from build123d import *

# Parameters (mm, degrees)
F0_W     = 508
F0_H     = 622.3
F0_W_2   = 68
F0_H_2   = 50.8
F1_DEPTH = 25.4
F2_DEPTH = 12.7
F3_DEPTH = 6.35


with BuildPart() as f1:
    # F0 (on Front) → F1 (new body)
    with BuildSketch(Plane.XZ):
        with Locations((0, -2.179809)):
            Rectangle(F0_W, F0_H)
        with BuildLine():
            Line((-44.45, 99.420191), (-44.45, 137.520191))
            Line((-44.45, 137.520191), (44.45, 137.520191))
            Line((44.45, 137.520191), (44.45, 99.420191))
            Line((44.45, 99.420191), (25.4, 99.420191))
            ThreePointArc((25.4, 99.420191), (20.909872, 97.560319), (19.05, 93.070191))
            Line((19.05, 93.070191), (19.05, 42.270191))
            ThreePointArc((19.05, 42.270191), (20.909872, 37.780063), (25.4, 35.920191))
            Line((25.4, 35.920191), (44.45, 35.920191))
            Line((44.45, 35.920191), (44.45, -2.179809))
            Line((44.45, -2.179809), (-44.45, -2.179809))
            Line((-44.45, -2.179809), (-44.45, 35.920191))
            Line((-44.45, 35.920191), (-25.4, 35.920191))
            ThreePointArc((-25.4, 35.920191), (-20.909872, 37.780063), (-19.05, 42.270191))
            Line((-19.05, 42.270191), (-19.05, 93.070191))
            ThreePointArc((-19.05, 93.070191), (-20.909872, 97.560319), (-25.4, 99.420191))
            Line((-25.4, 99.420191), (-44.45, 99.420191))
        make_face(mode=Mode.SUBTRACT)
        with Locations((0.576081, 175.620191)):
            Rectangle(F0_W_2, F0_H_2, mode=Mode.SUBTRACT)
    extrude(amount=F1_DEPTH)

    # F0 (on Front) → F2 (join)
    with BuildSketch(Plane.XZ):
        with Locations((0.576081, 175.620191)):
            Rectangle(F0_W_2, F0_H_2)
        Polygon((44.45, 137.520191), (-44.45, 137.520191), (-44.45, 99.420191), (-25.4, 99.420191), (25.4, 99.420191), (44.45, 99.420191), align=None)
        Polygon((25.4, 35.920191), (-25.4, 35.920191), (-44.45, 35.920191), (-44.45, -2.179809), (44.45, -2.179809), (44.45, 35.920191), align=None)
    extrude(amount=F2_DEPTH)

    # F0 (on Front) → F3 (join)
    with BuildSketch(Plane.XZ):
        with BuildLine():
            Line((25.4, 99.420191), (-25.4, 99.420191))
            ThreePointArc((-25.4, 99.420191), (-20.909872, 97.560319), (-19.05, 93.070191))
            Line((-19.05, 93.070191), (-19.05, 42.270191))
            ThreePointArc((-19.05, 42.270191), (-20.909872, 37.780063), (-25.4, 35.920191))
            Line((-25.4, 35.920191), (25.4, 35.920191))
            ThreePointArc((25.4, 35.920191), (20.909872, 37.780063), (19.05, 42.270191))
            Line((19.05, 42.270191), (19.05, 93.070191))
            ThreePointArc((19.05, 93.070191), (20.909872, 97.560319), (25.4, 99.420191))
        make_face()
    extrude(amount=F3_DEPTH)


solid = f1.part
For this review, take the finished solid that the model builds, in its own axes (mm). A direction names the side the tool comes from. Coordinates: 2 decimals unless noted, no trailing zeros. Loops run counter-clockwise (first coordinate to the right, second up) from the corner with the lowest first, then second, coordinate; pieces in that order, holes last. Notation, with made-up numbers: (7, -11) -> (63, -11) arc R24 cw to (63, 15) -> close; hole circle Ø9 at (-20.5, -3). An arc over 180 degrees is marked (long way). Write each question's results on one line, items separated by ' | '.
Q1. Mouldability with a two-part tool opening along Z and no side actions: class faces 1 (the flat face through (-254, -13, -7)), 2 (the flat face through (-4, -13, 308.97)), 3 (the flat face through (44.45, -19, 17)) as +Z half, -Z half, draft (parallel to the pull), parting line (faces both ways), or undercut.
Taken from the geometry:
face 1: draft | face 2: +Z half | face 3: undercut
Q2. To check wall thickness, follow line 1 along Z through (x, y) = (-12, -13.75); line 2 along X through (y, z) = (-20.5, 176); line 3 along X through (y, z) = (-14, 61). State the ranges of each line that lie inside material, in increasing order. Write a range as [from, to].
Taken from the geometry:
line 1: [-313.33, -2.18], [137.52, 150.22], [201.02, 308.97] | line 2: [-254, -33.42], [34.58, 254] | line 3: [-254, -19.05], [19.05, 254]
Q3. For pin 1 Ø5 at (x, z) = (-16, 100) entering from +Y, flat-tipped, find the tip position at first contact; note if it passes through.
Taken from the geometry:
pin 1: y = 0
Q4. Machinability: for faces 4 (the flat face through (-1, -12.7, 119)), 5 (the flat face through (-4, 0, 2)), which of the approach directions +Z, -Z, +X, -X, +Y, -Y give a long, thin tool a straight path to every point of the face, cutting with its end or side? Answer none if there is none.
Taken from the geometry:
face 4: -Y | face 5: +Z, -Z, +X, -X, +Y
Q5. Add section A-A, the plane y = -18. State the section outline as (x, z) points, then the cut area to 3 significant figures.
Taken from the geometry:
outline: (-254, -313.33) -> (254, -313.33) -> (254, 308.97) -> (-254, 308.97) -> close; hole (-44.45, -2.18) -> (44.45, -2.18) -> (44.45, 35.92) -> (25.4, 35.92) arc R6.35 cw to (19.05, 42.27) -> (19.05, 93.07) arc R6.35 cw to (25.4, 99.42) -> (44.45, 99.42) -> (44.45, 137.52) -> (-44.45, 137.52) -> (-44.45, 99.42) -> (-25.4, 99.42) arc R6.35 cw to (-19.05, 93.07) -> (-19.05, 42.27) arc R6.35 cw to (-25.4, 35.92) -> (-44.45, 35.92) -> close; hole (-33.42, 150.22) -> (34.58, 150.22) -> (34.58, 201.02) -> (-33.42, 201.02) -> close | area: 303,000 mm²
Q6. Add section B-B, the plane z = 85. State the section outline as (x, y) points.
Taken from the geometry:
outline: (-254, -25.4) -> (-19.05, -25.4) -> (-19.05, -6.35) -> (19.05, -6.35) -> (19.05, -25.4) -> (254, -25.4) -> (254, 0) -> (-254, 0) -> close
